Source: CAD feature listing. Evaluate the final solid. Frame: model axes, mm. Face numbers are marked on the shaded views. Give positions to 0.01 mm unless a question says otherwise; leave off trailing zeros. Order: outer loops, then holes, each group sorted by start corner. A loop starts at its lowest first (then second) coordinate and runs counter-clockwise, first axis right, second up.
1) Draft query along Y for the marked faces 1, 2, 3 and 4. Return one class per face: released by +Y, released by -Y, zero draft, split by the parting line, or undercut.
2) First-contact query: P1, Ø2, axis at x = 2, z = 1.5, coming from the +Y side (3 decimals); P2, Ø1.5, axis at x = 4, z = 0, coming from the -Y side. Flat tips, straight axial feed; report the tip coordinate or a pass-through.
3) Material intervals for line 1 (X direction, y = -1, z = 1); line 2 (X direction, y = -1.75, z = 1); line 3 (X direction, y = -6, z = -2.25), sorted ascending.
4) Section A-A, the plane z = -1.25. Return loops of the section in (x, y), plus the area to 3 significant figures.
```python
from build123d import *

# Parameters (mm, degrees)
SKETCH1_R         = 3.96875
EXTRUDE1_DEPTH    = 3.3734375
SKETCH7_OUTSIDE_W = 106.796
SKETCH7_OUTSIDE_H = 108.76
SKETCH7_OUTSIDE_R = 6.35
EXTRUDE2_DEPTH    = 25.4
EXTRUDE2_DRAFT    = -60


with BuildPart() as part:
    # Sketch1 → Extrude1 (new, symmetric)
    with BuildSketch(Plane.XY):
        Polygon((-6.35, 3.666174209), (-6.35, -3.666174209), (0, -7.332348419), (6.35, -3.666174209), (6.35, 3.666174209), (0, 7.332348419), align=None)
        Circle(SKETCH1_R, mode=Mode.SUBTRACT)
    extrude(amount=EXTRUDE1_DEPTH, both=True)


with BuildPart() as extrude2_tool:
    # Sketch7 outside → Extrude2 (with draft: the straight prism first)
    with BuildSketch(Plane.XY.offset(3.3734375)):
        Rectangle(SKETCH7_OUTSIDE_W, SKETCH7_OUTSIDE_H)
        Circle(SKETCH7_OUTSIDE_R, mode=Mode.SUBTRACT)
    extrude(amount=-EXTRUDE2_DEPTH)
    # Extrude2: the draft: its side faces are tilted about the plane it starts from
    extrude2_sides = [extrude2_tool.faces().sort_by_distance(p)[0] for p in [
        (0, -54.38, -9.3265625),
        (53.398, 0, -9.3265625),
        (0, 54.38, -9.3265625),
        (-53.398, 0, -9.3265625),
        (-6.35, 0, -9.3265625),
    ]]
    draft(extrude2_sides, Plane.XY.offset(3.3734375), EXTRUDE2_DRAFT)


with BuildPart() as part_1:
    add(part.part)

    # Extrude2: cut by extrude2_tool
    add(extrude2_tool.part, mode=Mode.SUBTRACT)


solid = part_1.part
```
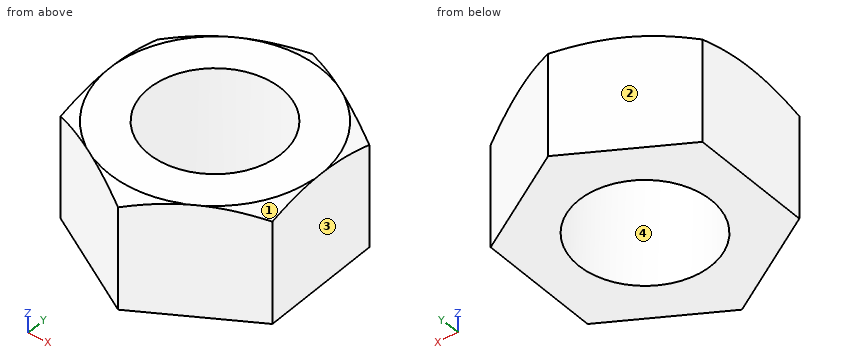
From the geometry:
1. face 1: released by -Y
1. face 2: released by +Y
1. face 3: zero draft
1. face 4: undercut
2. P1: stops at y = 6.755
2. P2: stops at y = -5.46
3. line 1: x = -6.35 to -3.84, 3.84 to 6.35
3. line 2: x = -6.35 to -3.56, 3.56 to 6.35
3. line 3: x = -2.31 to 2.31
4. outline: (-6.35, -3.67) - (0, -7.33) - (6.35, -3.67) - (6.35, 3.67) - (0, 7.33) - (-6.35, 3.67) - close; hole circle Ø7.94 at (0, 0)
4. area: 90.2 mm2
